Read the model definition and answer for the solid it produces. Units are mm, in the model's axes. Face numbers are marked on the shaded views. A direction names the side the tool comes from. Give positions to 0.01 mm unless a question says otherwise; leave off trailing zeros. Loops run counter-clockwise (first coordinate to the right, second up) from the corner with the lowest first, then second, coordinate; pieces in that order, holes last.
(1) Determine the mould class of the marked faces 1, 2 and 3 for opening direction X: pulls with the +X half, pulls with the -X half, needs draft (parallel to the pull), parting line crosses it, or undercut.
(2) Find section A-A, the plane x = -6. Write down the section's boundary in (y, z).
(3) Which of the six approach directions +Z, -Z, +X, -X, +Y, -Y give full straight-line access (tool end or side, diameter ignored) to the marked faces 4, 5, 6, 7 and 8?
(4) Each of these flat-tipped pins is pushed along its axis until it touches: P1, Ø2, axis at x = 2.5, y = -22.5, coming from the +Z side; P2, Ø12, axis at x = 27.5, z = -12.5, coming from the +Y side; P3, Ø12, axis at x = 9, y = -33, coming from the +Z side; P4, Ø0.8, axis at x = -39.5, y = -54.5, coming from the -Z side. Where does it stop, or does it pass through?
(5) Straight lines are drawn through the part: probe 1 along X at (y, z) = (-40, 10.5) (1 decimal); probe 2 along X at (y, z) = (-3.5, 1.5); probe 3 along Z at (x, y) = (-22.5, -9.5). For each, find the intervals that lie inside material, in ascending order.
Autodesk Inventor part; units mm, degrees
ref_plane "YZ Plane" through (0, 0, 0) normal (1, 0, 0) x (0, 1, 0)
ref_plane "XZ Plane" through (0, 0, 0) normal (0, 1, 0) x (-1, 0, 0)
ref_plane "XY Plane" through (0, 0, 0) normal (0, 0, 1) x (1, 0, 0)
sketch "Sketch1" plane through (0, 0, 0) normal (0, 1, 0) x (-1, 0, 0)
  line L0 (-40.259, 19.431) -> (40.259, 19.431)
  line L1 (40.259, 19.431) -> (40.259, -19.431)
  line L2 (40.259, -19.431) -> (-40.259, -19.431)
  line L3 (-40.259, -19.431) -> (-40.259, 19.431)
  line L4 (-40.259, 11.811) -> (-38.735, 11.811)
  line L5 (-38.735, 11.811) -> (-38.735, 10.287)
  line L6 (-38.735, 10.287) -> (-40.259, 10.287)
  line L7 (-40.259, 10.287) -> (-40.259, 11.811)
  line L8 (40.259, 11.811) -> (38.735, 11.811)
  line L9 (38.735, 11.811) -> (38.735, 10.287)
  line L10 (38.735, 10.287) -> (40.259, 10.287)
  line L11 (40.259, 10.287) -> (40.259, 11.811)
  point P0 (0, 0)
  point P1 (40.259, 0)
  point P2 (0, -19.431)
  point P3 (0, 0)
  dimension "d0" = 80.518
  dimension "d1" = 38.862
  dimension "d20" = 1.524
  dimension "d21" = 7.62
extrude "Extrusion1" add sketch "Sketch1" against normal blind 80.518 contours L0 L1 L8 L9 L10 L2 L3 L6 L5 L4
sketch "Sketch2" plane through (0, 0, 0) normal (0, 1, 0) x (-1, 0, 0)
  line L0 (-30.48, -11.811) -> (30.48, -11.811)
  line L1 (30.48, -11.811) -> (30.48, 11.811)
  line L2 (30.48, 11.811) -> (-30.48, 11.811)
  line L3 (-30.48, 11.811) -> (-30.48, -11.811)
  line L4 (40.259, -19.431) -> (-40.259, -19.431)
  line L5 (-40.259, 19.431) -> (40.259, 19.431)
  point P0 (0, 0)
  point P1 (0, 11.811)
  point P2 (-30.48, 0)
  dimension "d4" = 60.96
  dimension "d5" = 23.622
extrude "Extrusion2" cut sketch "Sketch2" against normal blind 14.478
sketch "Sketch3" plane through (0, -80.518, 0) normal (0, -1, 0) x (1, 0, 0)
  line L0 (-31.75, -12.7) -> (31.75, -12.7)
  line L1 (31.75, -12.7) -> (31.75, 12.7)
  line L2 (31.75, 12.7) -> (-31.75, 12.7)
  line L3 (-31.75, 12.7) -> (-31.75, -12.7)
  point P0 (0, 0)
  point P1 (0, -12.7)
  point P2 (-31.75, 0)
  dimension "d10" = 63.5
  dimension "d11" = 25.4
extrude "Extrusion3" cut sketch "Sketch3" against normal blind 14.478
sketch "Sketch4" plane through (40.259, 0, 19.431) normal (0, 0, 1) x (-1, 0, 0)
  line L0 (65.3415, 20.828) -> (15.1765, 20.828)
  line L1 (15.1765, 20.828) -> (15.1765, 61.214)
  line L2 (15.1765, 61.214) -> (65.3415, 61.214)
  line L3 (65.3415, 61.214) -> (65.3415, 20.828)
  line L4 (0, 0) -> (80.518, 0)
  point P0 (40.259, 0)
  point P1 (40.259, 0)
  point P2 (40.259, 20.828)
  dimension "d15" = 20.828
  dimension "d16" = 40.386
  dimension "d17" = 50.165
extrude "Extrusion4" cut sketch "Sketch4" against normal blind 27.178
fillet "Fillet1" radius 5.08 12 edges at (30.48, -7.239, 11.811) (30.48, -7.239, -11.811) (-30.48, -7.239, -11.811) (-30.48, -7.239, 11.811) (-31.75, -73.279, -12.7) (-31.75, -73.279, 12.7) (31.75, -73.279, 12.7) (31.75, -73.279, -12.7) (-25.0825, -20.828, 5.842) (25.0825, -20.828, 5.842) (25.0825, -61.214, 5.842) (-25.0825, -61.214, 5.842)
fillet "Fillet1" radius 7.62 4 edges at (-40.259, -40.259, 19.431) (-40.259, -40.259, -19.431) (40.259, -40.259, 19.431) (40.259, -40.259, -19.431)
fillet "Fillet2" radius 0.254 16 edges at (38.0273, -80.518, -17.1993) (0, -80.518, -19.431) (-38.0273, -80.518, -17.1993) (-40.259, -80.518, -0.7623) (40.259, -80.518, -0.7623) (0, -80.518, 19.431) (-38.0273, -80.518, 17.1993) (38.0273, -80.518, 17.1993) (0, 0, 19.431) (-38.0273, 0, 17.1993) (38.0273, 0, 17.1993) (38.0273, 0, -17.1993) (0, 0, -19.431) (-38.0273, 0, -17.1993) (-40.259, 0, -0.7623) (40.259, 0, -0.7623)
sketch "Sketch6" plane through (0, -14.478, 0) normal (0, 1, 0) x (1, 0, 0)
  line L0 (0, 27.2034) -> (0, -27.2034)
  line L1 (23.749, -11.811) -> (-23.749, -11.811)
  line L2 (-23.749, -11.811) -> (-23.749, 11.811)
  line L3 (-23.749, 11.811) -> (23.749, 11.811)
  line L4 (23.749, 11.811) -> (23.749, -11.811)
  line L5 (40.259, -10.287) -> (40.259, 11.811)
  line L6 (-40.259, 11.811) -> (-40.259, -10.287)
  line L7 (32.639, 19.431) -> (-32.639, 19.431)
  line L8 (25.4, -11.811) -> (-25.4, -11.811)
  line L9 (-25.4, 11.811) -> (25.4, 11.811)
  point P0 (0, 0)
  dimension "d26" = 16.51
  dimension "d28" = 16.51
  dimension "d30" = 0
  dimension "d31" = 0
extrude "Extrusion5" cut sketch "Sketch6" against normal blind 19.05
properties part number "Motor Passenger Section"
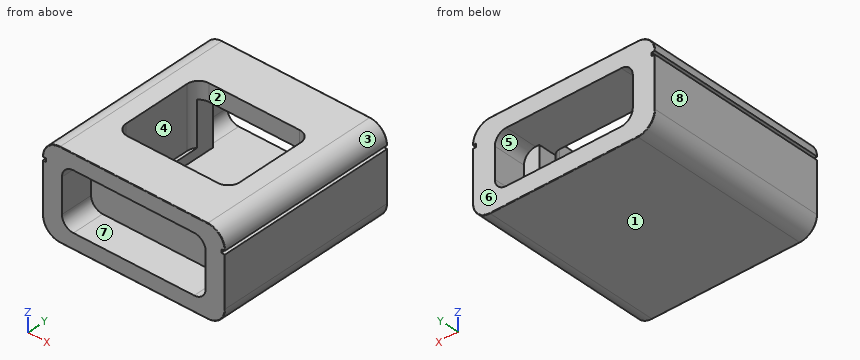
Entries:
1. face 1: needs draft
1. face 2: undercut
1. face 3: pulls with the +X half
2. outline: (-80.52, -19.18) arc R0.25 ccw to (-80.26, -19.43) - (-0.25, -19.43) arc R0.25 ccw to (0, -19.18) - (0, -11.81) - (-33.53, -11.81) - (-33.53, -7.75) - (-61.21, -7.75) - (-61.21, 19.43) - (-80.26, 19.43) arc R0.25 ccw to (-80.52, 19.18) - (-80.52, 12.7) - (-66.04, 12.7) - (-66.04, -12.7) - (-80.52, -12.7) - close; (-20.83, 11.81) - (0, 11.81) - (0, 19.18) arc R0.25 ccw to (-0.25, 19.43) - (-20.83, 19.43) - close
3. face 4: +Z
3. face 5: +Y
3. face 6: +Z, -Z, +X, -X, +Y
3. face 7: -Y
3. face 8: +Z, -Z, -X, +Y, -Y
4. P1: stops at z = -11.81
4. P2: stops at y = 0
4. P3: stops at z = -7.75
4. P4: stops at z = -15.85
5. probe 1: x = -38.7 to -25.1, 25.1 to 38.7
5. probe 2: x = -40.26 to -30.48, 30.48 to 40.26
5. probe 3: z = -19.43 to -11.81, 11.81 to 19.43
